Read the model definition and answer for the solid it produces. Units are mm, in the model's axes. Face numbers are marked on the shaded views. A direction names the side the tool comes from. Coordinates: 2 decimals unless noted, no trailing zeros. Order: outer loops, then holes, each group sorted by start corner. A loop starts at its lowest first (then second) coordinate and runs counter-clockwise, first axis right, second up. Notation, with made-up numbers: (85, 1) -> (100, 1) arc R15 cw to (100, 18) -> close; hole circle Ø8 at (-38.5, 66.25). An arc over 180 degrees is marked (long way). Return JSON: item names as keys, results as strings. Group by question number.
Autodesk Inventor part; units mm, degrees
ref_plane "YZ Plane" through (0, 0, 0) normal (1, 0, 0) x (0, 1, 0)
ref_plane "XZ Plane" through (0, 0, 0) normal (0, 1, 0) x (-1, 0, 0)
ref_plane "XY Plane" through (0, 0, 0) normal (0, 0, 1) x (1, 0, 0)
sketch "Sketch1" plane through (0, 0, 0) normal (0, 0, 1) x (1, 0, 0)
  line L0 (19, 0) -> (-19, 0)
  arc A0 (-9, 10) -> (-19, 0) centre (-9, 0) ccw
  line L1 (-9, 10) -> (68, 10)
  arc A1 (74, 4) -> (68, 10) centre (68, 4) ccw
  line L2 (74, 4) -> (74, -6.5)
  arc A2 (68, -12.5) -> (74, -6.5) centre (68, -6.5) ccw
  line L3 (68, -12.5) -> (51.8553, -12.5)
  arc A3 (51.8553, -12.5) -> (34.1777, -19.8223) centre (51.8553, -37.5) ccw
  line L4 (34.1777, -19.8223) -> (19, -35)
  line L5 (19, -35) -> (19, 0)
  line L6 (19, 0) -> (19, -22.9675) construction
  circle A4 centre (59, 2.5) radius 5.5
  point P0 (0, 0)
  point P1 (0, 0)
  dimension "d0" = 19
  dimension "d5" = 10
  dimension "d6" = 35
  dimension "d7" = 40
  dimension "d8" = 15
  dimension "d9" = 15
  dimension "d12" = 6
  dimension "d13" = 25
  dimension "d14" = 11
  dimension "d15" = 7.5
  dimension "d30" = 19
  dimension "d31" = 45
extrude "Extrusion1" add sketch "Sketch1" along normal blind 17.5 and the other way blind 52.5
sketch "Sketch3" plane through (-9, 10, 17.5) normal (0, 1, 0) x (1, 0, 0)
  circle A0 centre (9, 17.5) radius 3.75
  circle A1 centre (9, 17.5) radius 6
  dimension "d23" = 7.5
  dimension "d24" = 12
extrude "Extrusion3" cut sketch "Sketch3" against normal through all contours A0
chamfer "Chamfer1" distance 2.25 angle 45 1 edges at (-3.75, 10, 0)
sketch "Sketch5" plane through (-9, 10, 17.5) normal (0, 1, 0) x (1, 0, 0)
  line L0 (28, 70) -> (28, 0)
  line L1 (83, 70) -> (83, 0)
  line L2 (83, 70) -> (83, 0)
  line L3 (83, 70) -> (28, 70)
  line L4 (0, 70) -> (77, 70)
  line L5 (28, 0) -> (38, 0)
  line L6 (77, 0) -> (0, 0)
  line L7 (83, 70) -> (83, 0)
  line L8 (83, 35) -> (58, 35)
  arc A0 (58, 35) -> (38, 15) centre (58, 15) ccw
  line L9 (38, 15) -> (38, 0)
  line L10 (38, 0) -> (83, 0)
  point P0 (9, 17.5)
  dimension "d32" = 10
  dimension "d33" = 35
  dimension "d34" = 20
extrude "Extrusion4" cut sketch "Sketch5" against normal through all contours L9 A0 L8 L1 L10 L6
properties part number "kallax-irja-hook"
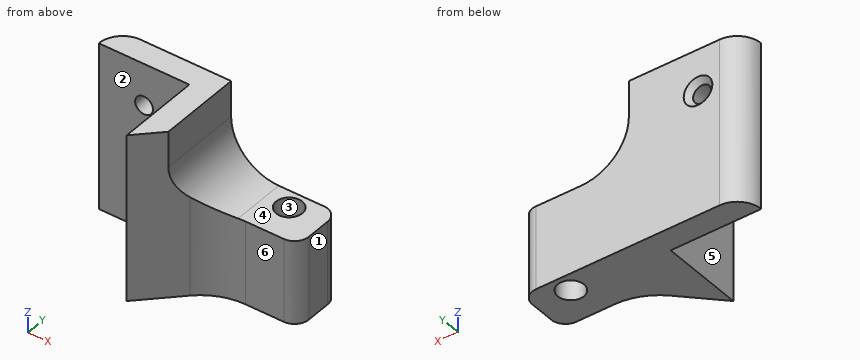
1. Given pin 1 (6 mm diameter, centred on x = 0, z = 0, fed in from +Y); pin 2 (11.5 mm diameter, centred on x = -6, z = -29, fed in from -Y); pin 3 (1 mm diameter, centred on y = -22.5, z = -14, fed in from +X); pin 4 (7 mm diameter, centred on x = 61, y = -2.5, fed in from +Z), each flat-ended and moving along its own axis, determine where each tip first touches the part or whether it passes through.
2. Straight lines are drawn through the part: L1, parallel to Z at x = 0, y = 2; L2, parallel to Y at x = 59, z = -37; L3, parallel to X at y = 5, z = 0. For each, find the intervals that lie inside material, in ascending order.
3. Find section D-D on y = -4. Determine the outline of the cut face in (x, z).
4. Find section B-B on x = 0. Determine the outline of the cut face in (y, z).
5. Find section C-C on z = -39. Determine the outline of the cut face in (x, y).
6. Which of the six approach directions +Z, -Z, +X, -X, +Y, -Y give full straight-line access (tool end or side, diameter ignored) to the marked faces 4, 5 and 6?
7. Find section A-A on y = 2.5. Determine the outline of the cut face in (x, z), and give its area (3 significant figures).
8. For a pull along X with two mould halves and no side action, classify the marked faces 1, 2 and 3 as released by +X, released by -X, zero draft, split by the parting line, or undercut.
Result:
{
 "1": {"pin 1": "through", "pin 2": "y = 0", "pin 3": "x = 32", "pin 4": "z = -17.5"},
 "2": {"L1": "-52.5 to -3.75, 3.75 to 17.5", "L2": "-12.5 to -3, 8 to 10", "L3": "-17.66 to -3.75, 3.75 to 29.16"},
 "3": {"outline": "(19, -52.5) -> (74, -52.5) -> (74, -17.5) -> (49, -17.5) arc R20 cw to (29, 2.5) -> (29, 17.5) -> (19, 17.5) -> close"},
 "4": {"outline": "(0, -52.5) -> (10, -52.5) -> (10, -6) -> (7.75, -3.75) -> (0, -3.75) -> close; (0, 3.75) -> (7.75, 3.75) -> (10, 6) -> (10, 17.5) -> (0, 17.5) -> close"},
 "5": {"outline": "(-19, 0) -> (19, 0) -> (19, -35) -> (34.18, -19.82) arc R25 cw to (51.86, -12.5) -> (68, -12.5) arc R6 ccw to (74, -6.5) -> (74, 4) arc R6 ccw to (68, 10) -> (-9, 10) arc R10 ccw to start; hole circle Ø11 at (59, 2.5)"},
 "6": {"face 4": "+Z, +X, +Y, -Y", "face 5": "+Z, -Z, -X, -Y", "face 6": "+Z, -Z, +X, -Y"},
 "7": {"outline": "(-18.68, -52.5) -> (53.5, -52.5) -> (53.5, -17.5) -> (49, -17.5) arc R20 cw to (29, 2.5) -> (29, 17.5) -> (-18.68, 17.5) -> close; (64.5, -52.5) -> (74, -52.5) -> (74, -17.5) -> (64.5, -17.5) -> close; hole circle Ø7.5 at (0, 0)", "area": "4,570 mm^2"},
 "8": {"face 1": "released by +X", "face 2": "zero draft", "face 3": "undercut"}
}
